Part model, mm, in its own coordinate system. Round coordinates to 2 decimals unless told otherwise and drop trailing zeros. Write each loop counter-clockwise with the first axis right and the second up, starting at its lowest first coordinate (ties: lowest second). Pieces come first, ordered by that corner, then holes. Notation, with made-up numbers: M 31,63.5 L 67,63.5 A18 cw 67,67.5 Z; hole C -25,42.25 d8. An arc over 180 degrees is marked long. Use a Markdown table: item, result. Add a question column.
1) Slice it at C-C on z = -0.7. Write the cut outline in (x, y).
2) Wall check: probe 1 along X at (y, z) = (0, -1.25); probe 2 along Y at (x, z) = (0, -0.35); probe 3 along Y at (x, z) = (0, -0.5) (3 decimals). Give the ranges that are in metal, low to high.
3) Drop flat-ended pins along their axis: P1, Ø2, axis at x = -67.5, z = -1, coming from the +Y side; P2, Ø4.5, axis at x = 0, y = 0, coming from the +Z side. Give the stop position or say it passes through.
4) Slice it at B-B on x = 0. Write the cut outline in (y, z) (3 decimals), plus the area to 3 significant figures.
5) Slice it at A-A on y = 0. Write the cut outline in (x, z), plus the area to 3 significant figures.
```python
from build123d import *

# Parameters (mm, degrees)
SKETCH1_W               = 200
SKETCH1_H               = 8
BOSS_EXTRUDE1_DEPTH     = 2.75
BEARING_CUTS_DEPTH      = 101.117743183
BEARING_CUTS_DEPTH_BACK = 101.117743183
SKETCH2_R               = 2.3


with BuildPart() as part:
    # Sketch1 → Boss-Extrude1 (new, symmetric)
    with BuildSketch(Plane.XY):
        Rectangle(SKETCH1_W, SKETCH1_H)
    extrude(amount=BOSS_EXTRUDE1_DEPTH, both=True)

    # Sketch2 → Bearing Cuts (cut, two sides: drawn at the far end of the back side and taken through both)
    with BuildSketch(Plane(origin=(0, 0, 0), x_dir=(0, 0, -1), z_dir=(1, 0, 0)).offset(-BEARING_CUTS_DEPTH_BACK)):
        with Locations((0, 4.5)):
            Circle(SKETCH2_R)
        with Locations((0, -4.5)):
            Circle(SKETCH2_R)
    extrude(amount=BEARING_CUTS_DEPTH + BEARING_CUTS_DEPTH_BACK, mode=Mode.SUBTRACT)

    # Sketch5 → CSK for M3 SFHCS1 (revolve, cut)
    with BuildSketch(Plane(origin=(0, 0, 2.75), x_dir=(0, -1, 0), z_dir=(1, 0, 0))):
        Polygon((0, 0), (0, 5.5), (2, 5.5), (1.7, 5.2), (1.7, 1.66), (3.36, 0), align=None)
    revolve(axis=Axis((0, 0, 9.1), (0, 0, -1)), mode=Mode.SUBTRACT)


solid = part.part
```
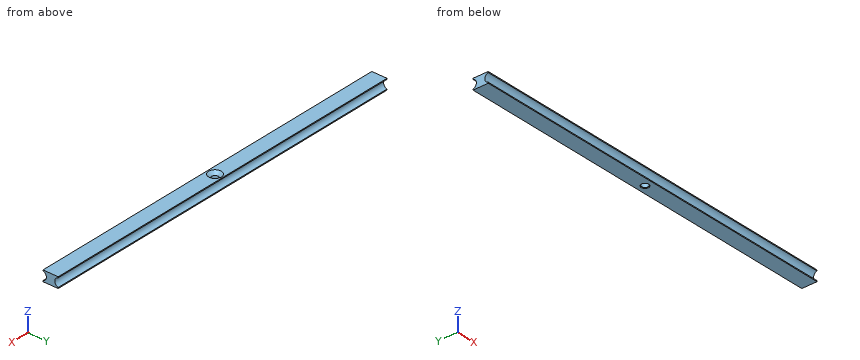
Entries:
| question | item | result |
|---|---|---|
| 1 | outline | M -100,-2.31 L 100,-2.31 L 100,2.31 L -100,2.31 Z; hole C 0,0 d3.4 |
| 2 | probe 1 | x = -100 to -1.7, 1.7 to 100 |
| 2 | probe 2 | y = -2.23 to -1.7, 1.7 to 2.23 |
| 2 | probe 3 | y = -2.255 to -1.7, 1.7 to 2.255 |
| 3 | P1 | stops at y = 3.36 |
| 3 | P2 | stops at z = 1.64 |
| 4 | outline | M -4,-2.75 L -2,-2.75 L -1.7,-2.45 L -1.7,1.09 L -3.36,2.75 L -4,2.75 L -4,2.245 A2.3 cw -4,-2.245 Z; M 1.7,-2.45 L 2,-2.75 L 4,-2.75 L 4,-2.245 A2.3 cw 4,2.245 L 4,2.75 L 3.36,2.75 L 1.7,1.09 Z |
| 4 | area | 10.4 mm^2 |
| 5 | outline | M -100,-2.75 L -2,-2.75 L -1.7,-2.45 L -1.7,1.09 L -3.36,2.75 L -100,2.75 Z; M 1.7,-2.45 L 2,-2.75 L 100,-2.75 L 100,2.75 L 3.36,2.75 L 1.7,1.09 Z |
| 5 | area | 1,080 mm^2 |
